Could you check a few things on this model? Use its own coordinates, in mm. A direction names the side the tool comes from. Give positions to 0.01 mm unless a question says otherwise; leave off trailing zeros. Order: outer loops, then holes, each group sorted by start corner. A loop starts at its lowest first (then second) coordinate and runs counter-clockwise, first axis right, second up. Notation, with made-up numbers: (62.25, 64) -> (81.25, 64) arc R8 cw to (81.25, 79) -> close; hole circle Ø9 at (64.5, 65.25). An arc over 180 degrees is marked (long way). Answer as CSV lines item,"result". Start each with the question number.
(1) I want a section at A-A (x = 0). Please give me the cut outline in (y, z), plus the area to 3 significant figures.
(2) I need wall thicknesses on L1, parallel to Y at x = 0.3, z = -63; L2, parallel to Y at x = -2.1, z = 25.5; L3, parallel to Z at x = 1.6, y = 19. Which ranges of each line are inside material? Lowest first, please.
(3) We'd pull the mould along Y, two halves only. Please class faces 3 (the face through (-1.34, -33.89, -44.12)), 4 (the face through (0, -36, -90)): released by +Y, released by -Y, zero draft, split by the parting line, or undercut.
(4) Will these pins go through, and if not, where does the flat tip stop? pin 1 Ø2 at (x, y) = (0, -26.5) entering from +Z; pin 2 Ø2 at (x, y) = (0, 17) entering from +Z.
(5) On a 3-axis mill with a long thin cutter (end or side, diameter ignored), from which of +Z, -Z, +X, -X, +Y, -Y can I reach the whole of each face in a straight line? I mean faces 1 (the face through (-0.54, 33.56, -44.12)), 2 (the face through (0, 36, -90)). Say none if no direction works.
(6) I want a section at B-B (z = -4.5). Please give me the cut outline in (x, y), plus the area to 3 significant figures.
```python
from build123d import *

# Parameters (mm, degrees)
SKETCH1_R           = 2.5
REVOLVE1_ANGLE      = 180
SKETCH1_2_R         = 2.5
BOSS_EXTRUDE1_DEPTH = 90
SKETCH2_R           = 2.5
BOSS_EXTRUDE2_DEPTH = 90
CHAMFER1_SIZE       = 0.5


with BuildPart() as part:
    # Sketch1 → Revolve1 (revolve)
    with BuildSketch(Plane.XY):
        with Locations((0, 36)):
            Circle(SKETCH1_R)
    revolve(axis=Axis((0, 0, 0), (1, 0, 0)), revolution_arc=REVOLVE1_ANGLE)

    # Sketch1<2> → Boss-Extrude1 (add)
    with BuildSketch(Plane.XY):
        with Locations((0, 36)):
            Circle(SKETCH1_2_R)
    extrude(amount=-BOSS_EXTRUDE1_DEPTH)

    # Sketch2 → Boss-Extrude2 (add)
    with BuildSketch(Plane(origin=(0, 0, 0), x_dir=(-1, 0, 0), z_dir=(0, 0, -1))):
        with Locations((0, -36)):
            Circle(SKETCH2_R)
    extrude(amount=BOSS_EXTRUDE2_DEPTH)

    # Chamfer1
    chamfer1_edges = [part.edges().sort_by_distance(p)[0] for p in [
        (2.5, -36, -90),
        (-2.5, 36, -90),
    ]]
    chamfer(chamfer1_edges, length=CHAMFER1_SIZE)


solid = part.part
```
Final values:
1,outline,"(-38.5, -89.5) -> (-38, -90) -> (-34, -90) -> (-33.5, -89.5) -> (-33.5, 0) arc R33.5 cw to (33.5, 0) -> (33.5, -89.5) -> (34, -90) -> (38, -90) -> (38.5, -89.5) -> (38.5, 0) arc R38.5 ccw to (-38.5, 0) -> close"
1,area,"1,460 mm²"
2,L1,"-38.48 to -33.52, 33.52 to 38.48"
2,L2,"-27.3 to -23.45, 23.45 to 27.3"
2,L3,"28.29 to 32.82"
3,face 3,"undercut"
3,face 4,"zero draft"
4,pin 1,"z = 28.84"
4,pin 2,"z = 35.02"
5,face 1,"-Z"
5,face 2,"-Z, +X, -X, +Y, -Y"
6,outline,"circle Ø5 at (0, -36); circle Ø5 at (0, 36)"
6,area,"39.3 mm²"
